Geometry: final body of the model. Coordinates: model frame, mm. A direction names the side the tool comes from. Give positions to 0.01 mm unless a question says otherwise; leave off trailing zeros. Write each loop counter-clockwise with the first axis right and the second up, starting at its lowest first coordinate (ties: lowest second). Pieces come first, ordered by that corner, then holes. Notation, with made-up numbers: (-38, 1.5) -> (-7, 1.5) arc R28 ccw to (-7, 28.5) -> close; hole circle Ø7 at (-20, 28.25). An arc over 180 degrees is marked (long way). Answer in a Markdown table with one row per item. Add a question column.
from build123d import *

# Parameters (mm, degrees)
SKETCH_1_R      = 8
EXTRUDE_1_DEPTH = 2
SKETCH_2_R      = 2
EXTRUDE_2_DEPTH = 5
SKETCH_3_W      = 40
SKETCH_3_H      = 40
EXTRUDE_3_DEPTH = 3


with BuildPart() as part:
    # 草图1 → 凸台-拉伸1 (new body)
    with BuildSketch(Plane(origin=(0, 0, 0), x_dir=(1, 0, 0), z_dir=(0, 1, 0))):
        with Locations(Location((0, 0, 0), (0, 0, 270))):
            Circle(SKETCH_1_R)
    extrude(amount=EXTRUDE_1_DEPTH)

    # 草图2 → 凸台-拉伸2 (add)
    with BuildSketch(Plane(origin=(0, 2, 0), x_dir=(1, 0, 0), z_dir=(0, 1, 0))):
        with Locations(Location((0, 0, 0), (0, 0, 270))):
            Circle(SKETCH_2_R)
    extrude(amount=EXTRUDE_2_DEPTH)

    # 草图3 → 凸台-拉伸3 (add)
    with BuildSketch(Plane(origin=(0, 7, 0), x_dir=(1, 0, 0), z_dir=(0, 1, 0))):
        Rectangle(SKETCH_3_W, SKETCH_3_H)
    extrude(amount=EXTRUDE_3_DEPTH)


solid = part.part
Q1. Section D-D on x = 13.5. Return loops of the section in (y, z).
Q2. Contact query for flat-ended pins moving along their axis: pin 1 Ø12 at (x, z) = (9.5, -9) entering from -Y; pin 2 Ø1 at (x, z) = (12.5, 2.5) entering from -Y; pin 3 Ø3 at (y, z) = (2.5, 2) entering from +X. Output: stop coordinate, or through.
Q3. Line query: probe 1 along Y at (x, z) = (-6, 2); probe 2 along Y at (x, z) = (5, 14); probe 3 along X at (y, z) = (3.75, 0). Output: solid intervals per line, ascending. Write a range as from..to.
Q4. Access query for faces 5 (the cylindrical face through (-7.81, 0.99, -1.73)), 6 (the flat face through (-20, 8, 0)). Directions: +Z, -Z, +X, -X, +Y, -Y. A direction counts if a zero-diameter tool reaches every point of the face in a straight line with its end or side. Return the directions, or none.
Q5. Section B-B on z = 0. Return loops of the section in (x, y), and give its area (3 significant figures).
Q6. Section A-A on x = 6. Return loops of the section in (y, z).
Q7. Section C-C on y = 4. Return loops of the section in (x, z).
Q8. Pull-direction query (Y, two-part tool) for faces 1 (the flat face through (-2, 2, 2)), 2 (the flat face through (0, 8, -20)), 3 (the flat face through (0, 0, 0)), 4 (the cylindrical face through (-2, 4, 0)); classes: +Y half, -Y half, draft (parallel to the pull), parting line (faces both ways), or undercut.
Checks:
| question | item | result |
|---|---|---|
| 1 | outline | (7, -20) -> (10, -20) -> (10, 20) -> (7, 20) -> close |
| 2 | pin 1 | y = 0 |
| 2 | pin 2 | y = 7 |
| 2 | pin 3 | x = 7.98 |
| 3 | probe 1 | 0..2, 7..10 |
| 3 | probe 2 | 7..10 |
| 3 | probe 3 | -2..2 |
| 4 | face 5 | -Y |
| 4 | face 6 | +Z, -Z, -X, +Y, -Y |
| 5 | outline | (-20, 7) -> (-2, 7) -> (-2, 2) -> (-8, 2) -> (-8, 0) -> (8, 0) -> (8, 2) -> (2, 2) -> (2, 7) -> (20, 7) -> (20, 10) -> (-20, 10) -> close |
| 5 | area | 172 mm^2 |
| 6 | outline | (0, -5.29) -> (2, -5.29) -> (2, 5.29) -> (0, 5.29) -> close; (7, -20) -> (10, -20) -> (10, 20) -> (7, 20) -> close |
| 7 | outline | circle Ø4 at (0, 0) |
| 8 | face 1 | undercut |
| 8 | face 2 | draft |
| 8 | face 3 | -Y half |
| 8 | face 4 | undercut |
